Read the model definition and answer for the solid it produces. Units are mm, in the model's axes. Face numbers are marked on the shaded views. A direction names the side the tool comes from. Coordinates: 2 decimals unless noted, no trailing zeros. Order: outer loops, then holes, each group sorted by start corner. A loop starts at its lowest first (then second) coordinate and runs counter-clockwise, first axis right, second up. Notation, with made-up numbers: (-34.75, 85) -> (-4.75, 85) arc R19 cw to (-4.75, 100) -> close; hole circle Ø4 at (39, -1.75). An arc over 180 degrees is marked (long way). Answer as a JSON object with one key per item and string values. Group by question number.
1) A tool of negligible diameter and unlimited length cuts with its end or side. For the marked faces 1 and 2, from which of +Z, -Z, +X, -X, +Y, -Y can it reach the whole face along a straight path? Write none if from no direction.
2) Section C-C on z = -8.75 is taken. Determine the outline of the cut face in (x, y).
3) Section A-A on x = -13.5 is taken. Determine the outline of the cut face in (y, z).
4) Section D-D on z = 10.5 is taken. Determine the outline of the cut face in (x, y).
5) Consider L1, parallel to X at y = 2.4, z = -10.5; L2, parallel to X at y = 2.8, z = -4.5; L3, parallel to Z at x = -0.5, y = 2.2. Determine where each line is inside the solid, lowest interval first.
6) Given pin 1 (3 mm diameter, centred on x = -3.5, z = -4, fed in from +Y), flat-ended and moving along its own axis, determine where the tip first touches the part or whether it passes through.
7) Section B-B on y = 2.4 is taken. Determine the outline of the cut face in (x, z).
from build123d import *

# Parameters (mm, degrees)
SKETCH_1_W          = 35.5
SKETCH_1_H          = 24
EXTRUDE_1_DEPTH     = 3
SKETCH_2_W          = 31.5
SKETCH_2_H          = 20
CUT_EXTRUDE_1_DEPTH = 2
SKETCH_3_R          = 0.55
CUT_EXTRUDE_2_DEPTH = 2


with BuildPart() as part:
    # 草图1 → 凸台-拉伸1 (new body)
    with BuildSketch(Plane(origin=(0, 0, 0), x_dir=(1, 0, 0), z_dir=(0, 1, 0))):
        Rectangle(SKETCH_1_W, SKETCH_1_H)
    extrude(amount=EXTRUDE_1_DEPTH)

    # 草图2 → 切除-拉伸1 (cut)
    with BuildSketch(Plane(origin=(0, 3, 0), x_dir=(1, 0, 0), z_dir=(0, 1, 0))):
        Rectangle(SKETCH_2_W, SKETCH_2_H)
    extrude(amount=-CUT_EXTRUDE_1_DEPTH, mode=Mode.SUBTRACT)

    # 草图3 → 切除-拉伸2 (cut)
    with BuildSketch(Plane(origin=(0, 3, 0), x_dir=(1, 0, 0), z_dir=(0, 1, 0))):
        with Locations(Location((-16.25, 10.5, 0), (0, 0, 270))):
            Circle(SKETCH_3_R)
        with Locations(Location((-16.25, -10.5, 0), (0, 0, 270))):
            Circle(SKETCH_3_R)
        with Locations(Location((16.25, -10.5, 0), (0, 0, 270))):
            Circle(SKETCH_3_R)
        with Locations(Location((16.25, 10.5, 0), (0, 0, 270))):
            Circle(SKETCH_3_R)
    extrude(amount=-CUT_EXTRUDE_2_DEPTH, mode=Mode.SUBTRACT)


solid = part.part
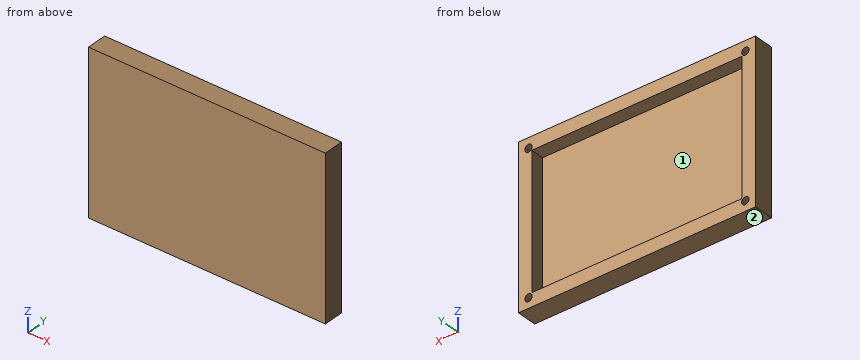
Worked answers:
{
 "1": {"face 1": "+Y", "face 2": "-Z, +X, -X, +Y, -Y"},
 "2": {"outline": "(-17.75, 0) -> (17.75, 0) -> (17.75, 3) -> (15.75, 3) -> (15.75, 1) -> (-15.75, 1) -> (-15.75, 3) -> (-17.75, 3) -> close"},
 "3": {"outline": "(0, -12) -> (3, -12) -> (3, -10) -> (1, -10) -> (1, 10) -> (3, 10) -> (3, 12) -> (0, 12) -> close"},
 "4": {"outline": "(-17.75, 0) -> (17.75, 0) -> (17.75, 3) -> (16.8, 3) -> (16.8, 1) -> (15.7, 1) -> (15.7, 3) -> (-15.7, 3) -> (-15.7, 1) -> (-16.8, 1) -> (-16.8, 3) -> (-17.75, 3) -> close"},
 "5": {"L1": "x = -17.75 to -16.8, -15.7 to 15.7, 16.8 to 17.75", "L2": "x = -17.75 to -15.75, 15.75 to 17.75", "L3": "z = -12 to -10, 10 to 12"},
 "6": {"pin 1": "stops at y = 1"},
 "7": {"outline": "(-17.75, -12) -> (17.75, -12) -> (17.75, 12) -> (-17.75, 12) -> close; hole circle Ø1.1 at (-16.25, -10.5); hole circle Ø1.1 at (-16.25, 10.5); hole (-15.75, -10) -> (15.75, -10) -> (15.75, 10) -> (-15.75, 10) -> close; hole circle Ø1.1 at (16.25, -10.5); hole circle Ø1.1 at (16.25, 10.5)"}
}
